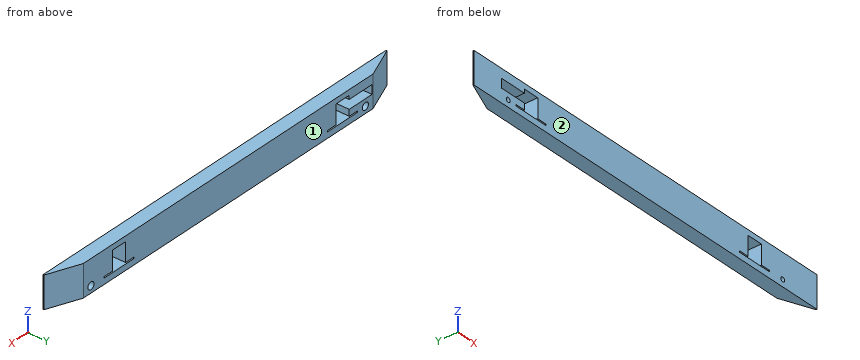
```python
from build123d import *

# Parameters (mm, degrees)
BOSS_EXTRUDE1_DEPTH             = 35
CUT_EXTRUDE1_DEPTH              = 452.608237303
CUT_EXTRUDE2_DEPTH              = 452.608237303
M8X1_0_TAPPED_HOLE1_D           = 5
M8X1_0_TAPPED_HOLE1_CBORE_D     = 8
M8X1_0_TAPPED_HOLE1_CBORE_DEPTH = 5


with BuildPart() as part:
    # Sketch1 → Boss-Extrude1 (new body)
    with BuildSketch(Plane.XY.offset(35)):
        Polygon((0, 0), (450, 0), (450, 1), (415, 15), (35, 15), (0, 1), align=None)
    extrude(amount=-BOSS_EXTRUDE1_DEPTH)

    # Sketch2 → Cut-Extrude1 (cut, through all)
    with BuildSketch(Plane(origin=(0, 15, 0), x_dir=(-1, 0, 0), z_dir=(0, 1, 0))):
        Polygon((-359.5, 8), (-359.5, 29.2), (-377, 29.2), (-377, 8), (-388, 8), (-388, 6.5), (-348.5, 6.5), (-348.5, 8), align=None)
    extrude(amount=-CUT_EXTRUDE1_DEPTH, mode=Mode.SUBTRACT)

    # Sketch3 → Cut-Extrude2 (cut, through all)
    with BuildSketch(Plane.XZ):
        Polygon((66.25, 15), (66.25, 8), (55.25, 8), (55.25, 6.5), (94.75, 6.5), (94.75, 8), (83.75, 8), (83.75, 29.2), (66.25, 29.2), (66.25, 25), (36.25, 25), (36.25, 15), align=None)
    extrude(amount=-CUT_EXTRUDE2_DEPTH, mode=Mode.SUBTRACT)

    # M8x1.0 Tapped Hole1 (through all)
    with Locations(Plane(origin=(0, 15, 0), x_dir=(1, 0, 0), z_dir=(0, 1, 0))):
        with Locations((45, -7.5), (405, -7.5)):
            CounterBoreHole(M8X1_0_TAPPED_HOLE1_D / 2, M8X1_0_TAPPED_HOLE1_CBORE_D / 2, M8X1_0_TAPPED_HOLE1_CBORE_DEPTH)


solid = part.part
```
Verification items for the finished model (mm, model axes). Face numbers are marked on the shaded views. Round coordinates to 2 decimals unless told otherwise and drop trailing zeros. Loops run counter-clockwise (first coordinate to the right, second up) from the corner with the lowest first, then second, coordinate; pieces in that order, holes last. Notation, with made-up numbers: (53.25, -20.5) -> (84.25, -20.5) arc R10 ccw to (84.25, -1.5) -> close; hole circle Ø2 at (-25, 79.5). An arc over 180 degrees is marked (long way). Answer as a JSON object with one key per item and string values.
Q1. Section check B-B (x = 60). Record the boundary of the cut face in (y, z).
Data:
{"outline": "(0, 0) -> (15, 0) -> (15, 6.5) -> (0, 6.5) -> close; (0, 8) -> (15, 8) -> (15, 15) -> (0, 15) -> close; (0, 25) -> (15, 25) -> (15, 35) -> (0, 35) -> close"}
Q2. Draft check along Y on the marked faces 1 and 2. Enter one of: pulls with the +Y half, pulls with the -Y half, needs draft (parallel to the pull), parting line crosses it, or undercut.
Data:
{"face 1": "pulls with the +Y half", "face 2": "pulls with the -Y half"}
Q3. Section check A-A (y = 4.5). Record the boundary of the cut face in (x, z), then the cut area to 3 significant figures.
Data:
{"outline": "(8.75, 0) -> (441.25, 0) -> (441.25, 35) -> (8.75, 35) -> close; hole (36.25, 15) -> (66.25, 15) -> (66.25, 8) -> (55.25, 8) -> (55.25, 6.5) -> (94.75, 6.5) -> (94.75, 8) -> (83.75, 8) -> (83.75, 29.2) -> (66.25, 29.2) -> (66.25, 25) -> (36.25, 25) -> close; hole circle Ø5 at (45, 7.5); hole (348.5, 6.5) -> (388, 6.5) -> (388, 8) -> (377, 8) -> (377, 29.2) -> (359.5, 29.2) -> (359.5, 8) -> (348.5, 8) -> close; hole circle Ø5 at (405, 7.5)", "area": "13,900 mm2"}
Q4. Scan lines: line 1 (X direction, y = 0.5, z = 29); line 2 (Z direction, x = 45, y = 11.75); line 3 (Z direction, x = 405, y = 13.55). Record each from-to range of solid material in increasing order. Write a range as from..to.
Data:
{"line 1": "x = 0..66.25, 83.75..359.5, 377..450", "line 2": "z = 0..3.5, 11.5..15, 25..35", "line 3": "z = 0..3.5, 11.5..35"}
Q5. Go/stop test with flat-tipped pins: P1, Ø9, axis at x = 405, z = 7.5, coming from the -Y side; P2, Ø5.5, axis at y = 4.5, z = 10, coming from the +X side (3 decimals); P3, Ø4.5, axis at y = 5.5, z = 19.5, coming from the -X side (3 decimals); P4, Ø3, axis at y = 12.5, z = 18, coming from the -X side. Record where each tip stops, or that it passes through.
Data:
{"P1": "stops at y = 0", "P2": "stops at x = 448.125", "P3": "stops at x = 5.625", "P4": "stops at x = 25"}
Q6. Section check C-C (z = 20.5). Record the boundary of the cut face in (x, y), then the cut area to 4 significant figures.
Data:
{"outline": "(0, 0) -> (36.25, 0) -> (36.25, 15) -> (35, 15) -> (0, 1) -> close; (83.75, 0) -> (359.5, 0) -> (359.5, 15) -> (83.75, 15) -> close; (377, 0) -> (450, 0) -> (450, 1) -> (415, 15) -> (377, 15) -> close", "area": "5,285 mm2"}
